Work out the finished part from the listing and answer in its coordinate system (mm). A direction names the side the tool comes from. Give positions to 0.01 mm unless a question says otherwise; leave off trailing zeros. Loops run counter-clockwise (first coordinate to the right, second up) from the corner with the lowest first, then second, coordinate; pieces in that order, holes last. Notation, with made-up numbers: M 6.25,8.5 L 51.25,8.5 A19 ccw 51.25,27.5 Z; hole C 41,12.25 d2. An arc over 180 degrees is marked long. Write item = value, one per line. Start each with the question number.
1. The mould has two halves that part along Y. Classify faces 1 (the face through (-17.452, -3.048, 7.395)), 2 (the face through (109, 240, 7)), 3 (the face through (-27.53, -179.16, 7.6)), 4 (the face through (140, -160, 7)): released by +Y, released by -Y, zero draft, split by the parting line, or undercut.
2. Consider L1, parallel to Y at x = 83, z = 1.75; L2, parallel to Y at x = 130, z = 5.5; L3, parallel to Y at x = -35.5, z = 1.75. Determine where each line is inside the solid, lowest interval first. Write a range as [from, to].
3. Section B-B on x = -33 is taken. Determine the outline of the cut face in (y, z).
4. Flat-ended cylindrical pins translate along their axes: pin 1 Ø4 at (x, y) = (-44.1, 124.1) entering from +Z; pin 2 Ø2 at (y, z) = (75.5, 9.5) entering from +X; pin 3 Ø8 at (y, z) = (135, 12.5) entering from -X; pin 4 Ø6 at (x, z) = (28, 2) entering from +Y. Find the tip coordinate at first contact, or state that the pin passes through.
5. For faces 5 (the face through (-87.96, -3.69, 0.99)), 6 (the face through (-26, 2, 0)), determine the directions among +Z, -Z, +X, -X, +Y, -Y from which every point of the face is accessible in a straight line to the end or side of a thin tool.
6. Section D-D on x = 16 is taken. Determine the outline of the cut face in (y, z).
7. Section C-C on z = 11.75 is taken. Give the number of separate pieces and of enclosed holes in the cut face, plus the area to 3 significant figures.
8. Section A-A on y = 0 is taken. Determine the outline of the cut face in (x, z), plus the area to 3 significant figures.
```python
from build123d import *

# Parameters (mm, degrees)
EXTRUDE_1_DEPTH          = 15
CUT_EXTRUDE_2_DEPTH      = 2
SKETCH_2_R               = 97.5
CUT_EXTRUDE_3_DEPTH      = 279.25348156
CUT_EXTRUDE_4_DEPTH      = 279.25348156
CUT_EXTRUDE_4_DEPTH_BACK = 279.25348156
HOLE_WIZARD_M6_1_D       = 5


with BuildPart() as part:
    # 草图1 → 凸台-拉伸1 (new body)
    with BuildSketch(Plane.XY):
        with BuildLine():
            Line((140, 183), (140, 240))
            Line((140, 240), (-140, 240))
            Line((-140, 240), (-140, -240))
            Line((-140, -240), (140, -240))
            Line((140, -240), (140, -183))
            Line((140, -183), (80, -183))
            ThreePointArc((80, -183), (-103, 0), (80, 183))
            Line((80, 183), (140, 183))
        make_face()
        with BuildLine():
            Line((140, -168), (140, 168))
            Line((140, 168), (80, 168))
            ThreePointArc((80, 168), (-88, 0), (80, -168))
            Line((80, -168), (140, -168))
        make_face()
        with BuildLine():
            Line((140, 168), (140, 183))
            Line((140, 183), (80, 183))
            ThreePointArc((80, 183), (-103, 0), (80, -183))
            Line((80, -183), (140, -183))
            Line((140, -183), (140, -168))
            Line((140, -168), (80, -168))
            ThreePointArc((80, -168), (-88, 0), (80, 168))
            Line((80, 168), (140, 168))
        make_face()
    extrude(amount=EXTRUDE_1_DEPTH)

    # 草图1<4> → 切除-拉伸2 (cut)
    with BuildSketch(Plane.XY):
        with BuildLine():
            Line((140, 168), (140, 183))
            Line((140, 183), (80, 183))
            ThreePointArc((80, 183), (-103, 0), (80, -183))
            Line((80, -183), (140, -183))
            Line((140, -183), (140, -168))
            Line((140, -168), (80, -168))
            ThreePointArc((80, -168), (-88, 0), (80, 168))
            Line((80, 168), (140, 168))
        make_face()
    extrude(amount=CUT_EXTRUDE_2_DEPTH, mode=Mode.SUBTRACT)

    # 草图2 → 切除-拉伸3 (cut, through all)
    with BuildSketch(Plane(origin=(0, 0, 0), x_dir=(-1, 0, 0), z_dir=(0, 0, -1))):
        with Locations((-80, 0)):
            Circle(SKETCH_2_R)
    extrude(amount=-CUT_EXTRUDE_3_DEPTH, mode=Mode.SUBTRACT)

    # 草图3 → 切除-拉伸4 (cut, two sides: drawn at the far end of the back side and taken through both)
    with BuildSketch(Plane(origin=(0, 0, 0), x_dir=(-1, 0, 0), z_dir=(0, 0, -1)).offset(-CUT_EXTRUDE_4_DEPTH_BACK)):
        Polygon((140, 240), (-77.846096908, 240), (130, 120), (130, -120), (-77.846096908, -240), (140, -240), align=None)
    extrude(amount=CUT_EXTRUDE_4_DEPTH + CUT_EXTRUDE_4_DEPTH_BACK, mode=Mode.SUBTRACT)

    # M6 螺纹孔1 (through all)
    with Locations(Plane(origin=(0, 0, 2), x_dir=(-1, 0, 0), z_dir=(0, 0, -1))):
        with Locations((-34.577257585, -169.519982514), (44.097240098, -124.097240098), (89.519982514, -45.422742415), (89.519982514, 45.422742415), (44.097240098, 124.097240098), (-34.577257585, 169.519982514), (-130, 175.5), (-130, -175.5)):
            Hole(HOLE_WIZARD_M6_1_D / 2)


solid = part.part
```
Verdict:
q1.face_1 = undercut
q1.face_2 = released by +Y
q1.face_3 = released by -Y
q1.face_4 = zero draft
q2.L1 = [-240, -183], [-168, -97.45], [97.45, 168], [183, 240]
q2.L2 = [-240, -178], [-173, -83.7], [83.7, 173], [178, 240]
q2.L3 = [-174.56, -141.95], [-122, 122], [141.95, 174.56]
q3.outline = M -176,0 L -143.94,0 L -143.94,2 L -124.32,2 L -124.32,0 L 124.32,0 L 124.32,2 L 143.94,2 L 143.94,0 L 176,0 L 176,15 L -176,15 Z
q4.pin_1 = through
q4.pin_2 = 19.55
q4.pin_3 = -110.95
q4.pin_4 = 212.95
q5.face_5 = -Z
q5.face_6 = -Z, +X, -X, +Y, -Y
q6.outline = M -204.29,0 L -171.44,0 L -171.44,2 L -155.33,2 L -155.33,0 L -73.55,0 L -73.55,15 L -204.29,15 Z; M 73.55,0 L 155.33,0 L 155.33,2 L 171.44,2 L 171.44,0 L 204.29,0 L 204.29,15 L 73.55,15 Z
q7.separate_pieces = 1
q7.enclosed_holes = 8
q7.area = 78,700 mm2
q8.outline = M -130,0 L -103,0 L -103,2 L -88,2 L -88,0 L -17.5,0 L -17.5,15 L -130,15 Z
q8.area = 1,660 mm2
